Here's how the part is built. I have some questions about the finished solid (model axes, mm). A direction names the side the tool comes from. Coordinates: 2 decimals unless noted, no trailing zeros. Order: outer loops, then holes, each group sorted by start corner. A loop starts at its lowest first (then second) coordinate and runs counter-clockwise, first axis right, second up. Notation, with made-up numbers: (-33, -18) - (-7, -18) arc R14 ccw to (-7, 5) - close; hole circle Ø7 at (81, -24). An arc over 180 degrees is marked (long way). Answer in a Markdown table with one row per item. Add a question column.
Item 1: On a 3-axis mill with a long thin cutter (end or side, diameter ignored), from which of +Z, -Z, +X, -X, +Y, -Y can I reach the whole of each face in a straight line? I mean faces 1 (the cylindrical face through (-1.72, 7.75, 3.13)), 2 (the flat face through (-3.8, 7.3, 0)). Say none if no direction works.
Item 2: Thinking about a two-plate mould opening in X: for faces 3 (the flat face through (3, 4, 15.875)), 4 (the cylindrical face through (-3.441, -15.497, 7.826)), 5 (the cylindrical face through (-3.78, 2.9, 11.05)), 6 (the flat face through (0, 5, 6.35)), which applies, +X half, -X half, draft (parallel to the pull), parting line (faces both ways), or undercut?
Item 3: I want a section at D-D (x = 12.5). Please give me the cut outline in (y, z) (3 decimals).
Item 4: If I drill on line 1 along Y through (x, z) = (0, 12.5) (1 decimal); line 2 along Y through (x, z) = (0, 2.5) (1 decimal); line 3 along X through (y, z) = (3, 6), over which ranges is the centre line in solid material (lowest first)? Write a range as from..to.
Item 5: Will these pins go through, and if not, where does the flat tip stop? pin 1 Ø5 at (y, z) = (12, 7) entering from +X; pin 2 Ø3 at (y, z) = (6, 14) entering from +X; pin 3 Ø14.5 at (x, y) = (0, 0) entering from -Z.
```python
from build123d import *

# Parameters (mm, degrees)
F0_R     = 15.875
F0_R_2   = 7.9375
F1_DEPTH = 15.875
F2_R     = 7.9375
F3_DEPTH = 6.35
F4_R     = 4.7625
F5_DEPTH = 25.4


with BuildPart() as f1:
    # F0 (on Top) → F1 (new body)
    with BuildSketch(Plane.XY):
        Circle(F0_R)
        Circle(F0_R_2, mode=Mode.SUBTRACT)
        Circle(F0_R_2)
    extrude(amount=F1_DEPTH)

    # F2 (on face) → F3 (cut)
    with BuildSketch(Plane(origin=(0, 0, 0), x_dir=(1, 0, 0), z_dir=(0, 0, -1))):
        Circle(F2_R)
    extrude(amount=-F3_DEPTH, mode=Mode.SUBTRACT)

    # F4 (on face) → F5 (cut)
    with BuildSketch(Plane(origin=(0, 0, 6.35), x_dir=(1, 0, 0), z_dir=(0, 0, -1))):
        Circle(F4_R)
    extrude(amount=-F5_DEPTH, mode=Mode.SUBTRACT)


solid = f1.part
```
Values follow:
| question | item | result |
|---|---|---|
| 1 | face 1 | -Z |
| 1 | face 2 | -Z, +X, -X, +Y, -Y |
| 2 | face 3 | draft |
| 2 | face 4 | parting line |
| 2 | face 5 | undercut |
| 2 | face 6 | undercut |
| 3 | outline | (-9.786, 0) - (9.786, 0) - (9.786, 15.875) - (-9.786, 15.875) - close |
| 4 | line 1 | y = -15.9..-4.8, 4.8..15.9 |
| 4 | line 2 | y = -15.9..-7.9, 7.9..15.9 |
| 4 | line 3 | x = -15.59..-7.35, 7.35..15.59 |
| 5 | pin 1 | stops at x = 12.72 |
| 5 | pin 2 | stops at x = 15.22 |
| 5 | pin 3 | stops at z = 6.35 |
